Source: three-view drawing plus pictorial views. Frame: mm from the lowest corner of the part. Coordinates: 2 decimals unless noted, no trailing zeros. Order: outer loops, then holes, each group sorted by start corner. A loop starts at its lowest first (then second) coordinate and runs counter-clockwise, first axis right, second up. Notation, with made-up numbers: M 7,44 L 65,44 A17 cw 65,77 Z; hole C 79.25,73.5 d6. An arc over 180 degrees is marked long. Use CSV: the item, a comma, the result in double quotes. Start each with the question number.
Q1. Section query C-C, the plane z = 7.75. Output: boundary loops of the cut face in (x, y).
Q2. Section query B-B, the plane x = 77. Output: boundary loops of the cut face in (y, z), and give its area (3 significant figures).
Q3. Section query A-A, the plane y = 2. Output: boundary loops of the cut face in (x, z), and give its area (3 significant figures).
Q4. Ray query, probe 1 along X at (y, z) = (2, 6.25); probe 2 along X at (y, z) = (1.25, 4.75) (1 decimal); probe 3 along Z at (x, y) = (75, 5.5). Return the intervals inside material, ascending.
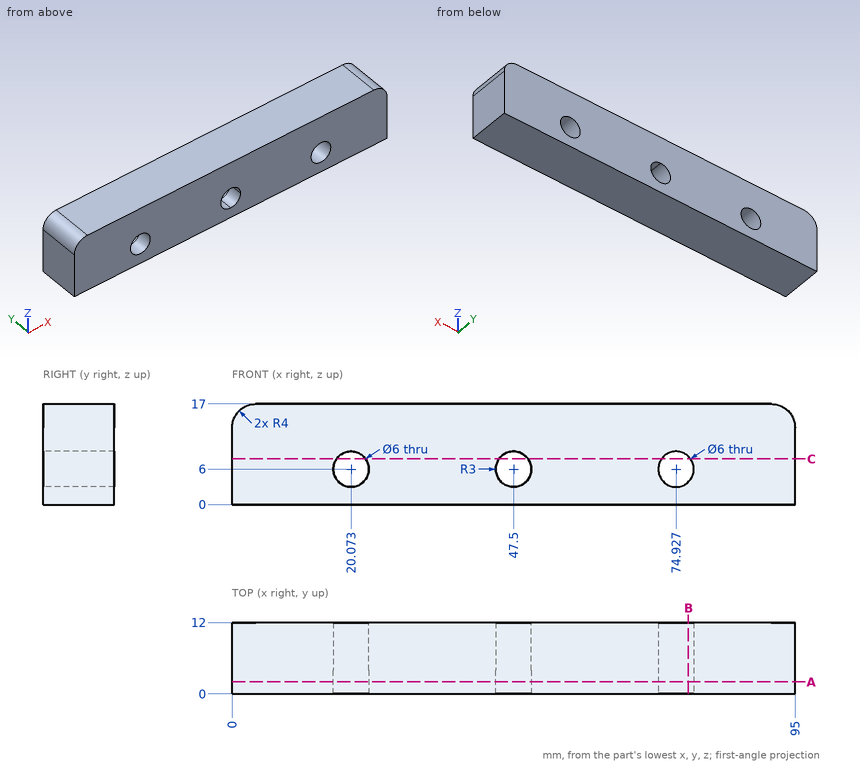
Responses:
1,outline,"M 0,0 L 17.64,0 L 17.64,12 L 0,12 Z; M 22.51,0 L 45.06,0 L 45.06,12 L 22.51,12 Z; M 49.94,0 L 72.49,0 L 72.49,12 L 49.94,12 Z; M 77.36,0 L 95,0 L 95,12 L 77.36,12 Z"
2,outline,"M 0,0 L 12,0 L 12,3.83 L 0,3.83 Z; M 0,8.17 L 12,8.17 L 12,17 L 0,17 Z"
2,area,"152 mm²"
3,outline,"M 0,0 L 95,0 L 95,13 A4 ccw 91,17 L 4,17 A4 ccw 0,13 Z; hole C 20.07,6 d6; hole C 47.5,6 d6; hole C 74.93,6 d6"
3,area,"1,520 mm²"
4,probe 1,"x = 0 to 17.08, 23.06 to 44.51, 50.49 to 71.94, 77.92 to 95"
4,probe 2,"x = 0 to 17.3, 22.8 to 44.8, 50.2 to 72.2, 77.7 to 95"
4,probe 3,"z = 0 to 3, 9 to 17"
